The model under review builds one solid part; all positions refer to its coordinate system, in mm. Face numbers are marked on the shaded views. A direction names the side the tool comes from. Coordinates: 2 decimals unless noted, no trailing zeros. Order: outer loops, then holes, each group sorted by start corner. A loop starts at its lowest first (then second) coordinate and runs counter-clockwise, first axis right, second up. Notation, with made-up numbers: (14.5, -8) -> (22.5, -8) arc R7 cw to (22.5, 3) -> close; hole circle Ø1 at (25, -33.5). An arc over 180 degrees is marked (long way). Use one line per item in the form item = value. Start each with the question number.
(1) Wall thickness on line 1 along Z through (x, y) = (-75, -2115); line 2 along Z through (x, y) = (75, 5); line 3 along Y through (x, z) = (-49, -84): over which ranges is each line inside the solid? List them lowest first.
(2) Take a section at B-B (z = 31.5). State the section outline as (x, y) points.
(3) Take a section at A-A (x = 41.5). State the section outline as (y, z) points.
(4) For the marked faces 1 and 2, list the 3-axis set-ups (+Z, -Z, +X, -X, +Y, -Y) from which the entire face can be reached by the end or side of a thin tool; tool diameter is ignored.
(5) Insertion check: pin 1 Ø4 at (y, z) = (-1367.5, -60.5) entering from -X; pin 2 Ø1 at (y, z) = (-553, 25.5) entering from +X; pin 3 Ø24 at (x, y) = (83, -55) entering from -Z; pin 4 Ø15.5 at (x, z) = (-75, 75) entering from -Y. Each pin has a flat end and moves straight along its axis. Give the tip position at first contact, or say it passes through.
(6) Take a section at C-C (y = -1311). State the section outline as (x, z) points, then the cut area to 3 significant figures.
```python
from build123d import *

# Parameters (mm, degrees)
F0_R          = 70
F0_R_2        = 65
F1_DEPTH      = 2110
F2_W          = 200
F2_H          = 200
F2_R          = 11
F3_DEPTH      = 10
F4_W          = 30.1787997812
F4_H          = 10
F4_W_2        = 10
F4_H_2        = 30.1787997812
F5_DEPTH      = 150
F6_T1_DEPTH   = 269.311363913
F6_T3_DEPTH   = 269.311363913
F6_T8_DEPTH   = 269.311363913
F6_S9_R       = 70
F6_T10_DEPTH  = 139
F8_W          = 200
F8_H          = 200
F8_R          = 8.5
F9_DEPTH      = 10
F10_W         = 10
F10_H         = 30.1787997812
F10_W_2       = 30.1787997812
F10_H_2       = 10
F11_DEPTH     = 80
F12_T1_DEPTH  = 269.311363913
F12_T3_DEPTH  = 269.311363913
F12_T8_DEPTH  = 269.311363913
F12_S9_R      = 70
F12_T10_DEPTH = 139
F12_T14_DEPTH = 269.311363913
F12_S15_R     = 70
F12_T16_DEPTH = 139


# Not quite as in the source:
# - a fillet or chamfer that OpenCascade refuses, or shapes differently, is made with other operations: its cross-section is extruded or revolved along the edge and cut away or added


with BuildPart() as f1:
    # F0 (on Front) → F1 (new body)
    with BuildSketch(Plane.XZ):
        Circle(F0_R)
        Circle(F0_R_2, mode=Mode.SUBTRACT)
    extrude(amount=F1_DEPTH)

    # F2 (on Front) → F3 (join)
    with BuildSketch(Plane.XZ):
        Rectangle(F2_W, F2_H)
        with Locations((-75, -75)):
            Circle(F2_R, mode=Mode.SUBTRACT)
        with Locations((75, -75)):
            Circle(F2_R, mode=Mode.SUBTRACT)
        with Locations((-75, 75)):
            Circle(F2_R, mode=Mode.SUBTRACT)
        with Locations((75, 75)):
            Circle(F2_R, mode=Mode.SUBTRACT)
    extrude(amount=-F3_DEPTH)

    # F4 (on Front) → F5 (join)
    with BuildSketch(Plane.XZ):
        with Locations((-84.9106001094, 0)):
            Rectangle(F4_W, F4_H)
        with Locations((0, 84.9106001094)):
            Rectangle(F4_W_2, F4_H_2)
        with Locations((84.9106001094, 0)):
            Rectangle(F4_W, F4_H)
        with Locations((0, -84.9106001094)):
            Rectangle(F4_W_2, F4_H_2)
    extrude(amount=F5_DEPTH)

    # F6: chamfer of 50 x 20 on 4 edges, made by hand

    # F6_s2 → F6_t1 (cut)
    with BuildSketch(Plane.YZ.offset(-134.6556819565)):
        Polygon((-100, 100), (-150, 80), (-150, 100), align=None)
        Polygon((-100, -100), (-150, -80), (-150, -100), align=None)
    extrude(amount=F6_T1_DEPTH, mode=Mode.SUBTRACT)

    # F6_s4 → F6_t3 (cut)
    with BuildSketch(Plane.XY.offset(-134.6556819565)):
        Polygon((100, -100), (80, -150), (100, -150), align=None)
    extrude(amount=F6_T3_DEPTH, mode=Mode.SUBTRACT)


with BuildPart() as f6_tool6:
    # F6_s7 → F6_t8 (new body)
    with BuildSketch(Plane.XY.offset(134.6556819565)):
        Polygon((-100, -130), (-50, -150), (-100, -150), align=None)
    extrude(amount=-F6_T8_DEPTH)

    # F6_s9 → F6_t10 (cut, symmetric)
    with BuildSketch(Plane.XZ.offset(140)):
        Circle(F6_S9_R)
    extrude(amount=F6_T10_DEPTH, both=True, mode=Mode.SUBTRACT)


with BuildPart() as f1_1:
    add(f1.part)

    # F6_t5: cut F6_tool6
    add(f6_tool6.part, mode=Mode.SUBTRACT)

    # F8 (on offset) → F9 (join)
    with BuildSketch(Plane.XZ.offset(2110)):
        Rectangle(F8_W, F8_H)
        with Locations((-75, -75)):
            Circle(F8_R, mode=Mode.SUBTRACT)
        with Locations((75, -75)):
            Circle(F8_R, mode=Mode.SUBTRACT)
        with Locations((-75, 75)):
            Circle(F8_R, mode=Mode.SUBTRACT)
        with Locations((75, 75)):
            Circle(F8_R, mode=Mode.SUBTRACT)
    extrude(amount=F9_DEPTH)

    # F10 (on face) → F11 (join)
    with BuildSketch(Plane(origin=(0, -2110, 0), x_dir=(-1, 0, 0), z_dir=(0, 1, 0))):
        with Locations((0, 84.9106001094)):
            Rectangle(F10_W, F10_H)
        with Locations((84.9106001094, 0)):
            Rectangle(F10_W_2, F10_H_2)
        with Locations((0, -84.9106001094)):
            Rectangle(F10_W, F10_H)
        with Locations((-84.9106001094, 0)):
            Rectangle(F10_W_2, F10_H_2)
    extrude(amount=F11_DEPTH)

    # F12: chamfer of 20 x 50 on 4 edges, made by hand

    # F12_s2 → F12_t1 (cut)
    with BuildSketch(Plane.YZ.offset(-134.6556819565)):
        Polygon((-2080, 100), (-2030, 80), (-2030, 100), align=None)
    extrude(amount=F12_T1_DEPTH, mode=Mode.SUBTRACT)

    # F12_s4 → F12_t3 (cut)
    with BuildSketch(Plane.XY.offset(-134.6556819565)):
        Polygon((100, -2080), (80, -2030), (100, -2030), align=None)
    extrude(amount=F12_T3_DEPTH, mode=Mode.SUBTRACT)


with BuildPart() as f12_tool6:
    # F12_s7 → F12_t8 (new body)
    with BuildSketch(Plane.XY.offset(-134.6556819565)):
        Polygon((-100, -2050), (-50, -2030), (-100, -2030), align=None)
    extrude(amount=F12_T8_DEPTH)

    # F12_s9 → F12_t10 (cut, symmetric)
    with BuildSketch(Plane.XZ.offset(2040)):
        Circle(F12_S9_R)
    extrude(amount=F12_T10_DEPTH, both=True, mode=Mode.SUBTRACT)


with BuildPart() as f1_2:
    add(f1_1.part)

    # F12_t5: cut F12_tool6
    add(f12_tool6.part, mode=Mode.SUBTRACT)


with BuildPart() as f12_tool12:
    # F12_s13 → F12_t14 (new body)
    with BuildSketch(Plane.YZ.offset(134.6556819565)):
        Polygon((-2050, -100), (-2030, -50), (-2030, -100), align=None)
    extrude(amount=-F12_T14_DEPTH)

    # F12_s15 → F12_t16 (cut, symmetric)
    with BuildSketch(Plane.XZ.offset(2040)):
        Circle(F12_S15_R)
    extrude(amount=F12_T16_DEPTH, both=True, mode=Mode.SUBTRACT)


with BuildPart() as f1_3:
    add(f1_2.part)

    # F12_t11: cut F12_tool12
    add(f12_tool12.part, mode=Mode.SUBTRACT)


solid = f1_3.part
```
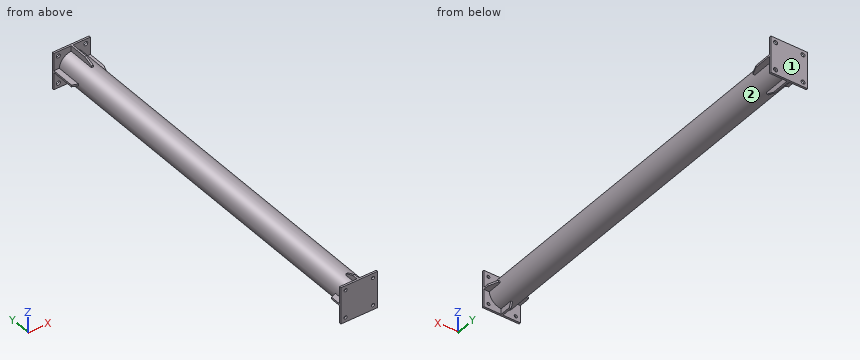
Findings:
q1.line_1 = -100 to -83.5, -66.5 to 66.5, 83.5 to 100
q1.line_2 = -100 to -86, -64 to 64, 86 to 100
q1.line_3 = -2120 to -2110, 0 to 10
q2.outline = (-100, -2120) -> (100, -2120) -> (100, -2110) -> (62.51, -2110) -> (62.51, 0) -> (100, 0) -> (100, 10) -> (-100, 10) -> (-100, 0) -> (-62.51, 0) -> (-62.51, -2110) -> (-100, -2110) -> close; hole (-56.86, -2110) -> (56.86, -2110) -> (56.86, 0) -> (-56.86, 0) -> close
q3.outline = (-2120, -100) -> (-2110, -100) -> (-2110, -56.37) -> (0, -56.37) -> (0, -100) -> (10, -100) -> (10, 100) -> (0, 100) -> (0, 56.37) -> (-2110, 56.37) -> (-2110, 100) -> (-2120, 100) -> close; hole (-2110, -50.03) -> (0, -50.03) -> (0, 50.03) -> (-2110, 50.03) -> close
q4.face_1 = +Z, -Z, +X, -X, +Y
q4.face_2 = none
q5.pin_1 = -38.44
q5.pin_2 = 65.38
q5.pin_3 = -5
q5.pin_4 = through
q6.outline = circle Ø140 at (0, 0); hole circle Ø130 at (0, 0)
q6.area = 2,120 mm²
